```python
from build123d import *

# Parameters (mm, degrees)
SKETCH1_R           = 9.36
SKETCH1_R_2         = 7.99
EXTRUDE1_DEPTH      = 670
SKETCH2_R           = 1.5
SKETCH2_R_2         = 5.5
EXTRUDE2_DEPTH      = 10.36
EXTRUDE2_DEPTH_BACK = 10.36
SKETCH3_W           = 7
SKETCH3_H           = 22
EXTRUDE3_DEPTH      = 25
EXTRUDE3_DEPTH_BACK = 25


with BuildPart() as part:
    # Sketch1 → Extrude1 (new body)
    with BuildSketch(Plane.XY):
        Circle(SKETCH1_R)
        Circle(SKETCH1_R_2, mode=Mode.SUBTRACT)
    extrude(amount=EXTRUDE1_DEPTH)

    # Sketch2 → Extrude2 (cut, two sides)
    with BuildSketch(Plane(origin=(0, 0, 0), x_dir=(0, 0, -1), z_dir=(1, 0, 0))) as extrude2_sk:
        with Locations((-30, 0)):
            Circle(SKETCH2_R)
        with Locations((-150, 0)):
            Circle(SKETCH2_R_2)
        with Locations((-136.0625, 0)):
            Circle(SKETCH2_R)
        with Locations((-163.9375, 0)):
            Circle(SKETCH2_R)
    extrude(amount=EXTRUDE2_DEPTH, mode=Mode.SUBTRACT)
    extrude(extrude2_sk.sketch, amount=-EXTRUDE2_DEPTH_BACK, mode=Mode.SUBTRACT)

    # Sketch3 → Extrude3 (cut, two sides)
    with BuildSketch(Plane(origin=(0, 0, 0), x_dir=(1, 0, 0), z_dir=(0, 1, 0))) as extrude3_sk:
        with Locations((0, -150)):
            Rectangle(SKETCH3_W, SKETCH3_H)
    extrude(amount=EXTRUDE3_DEPTH, mode=Mode.SUBTRACT)
    extrude(extrude3_sk.sketch, amount=-EXTRUDE3_DEPTH_BACK, mode=Mode.SUBTRACT)


solid = part.part
```
The model under review builds one solid part; all positions refer to its coordinate system, in mm. Round coordinates to 2 decimals unless told otherwise and drop trailing zeros. Order: outer loops, then holes, each group sorted by start corner. A loop starts at its lowest first (then second) coordinate and runs counter-clockwise, first axis right, second up. Notation, with made-up numbers: (30.5, -21) -> (48.5, -21) arc R17 ccw to (48.5, 9) -> close; hole circle Ø7 at (14, 58). An arc over 180 degrees is marked (long way). Use a Markdown table: item, result.
Q1. We need section B-B on z = 337. Write out the cut boundary in (x, y).
Values:
| item | result |
|---|---|
| outline | circle Ø18.72 at (0, 0); hole circle Ø15.98 at (0, 0) |
Q2. For line 1 (Z direction, x = 8.35, y = 0); line 2 (X direction, y = -0.25, z = 337.5); line 3 (Y direction, x = 3.25, z = 214.5), list the stretches that pass through material, from the lowest coordinate up.
Values:
| item | result |
|---|---|
| line 1 | z = 0 to 28.5, 31.5 to 134.56, 137.56 to 144.5, 155.5 to 162.44, 165.44 to 670 |
| line 2 | x = -9.36 to -7.99, 7.99 to 9.36 |
| line 3 | y = -8.78 to -7.3, 7.3 to 8.78 |
Q3. Clearance check with flat-ended pins moving along their axes: P1, Ø4, axis at x = -3, z = 553, coming from the +Y side; P2, Ø1.6, axis at y = 7.5, z = 153.5, coming from the +X side; P3, Ø1, axis at x = 6, z = 99.5, coming from the +Y side. State where each tip first meets the part, or that it passes through.
Values:
| item | result |
|---|---|
| P1 | stops at y = 9.31 |
| P2 | stops at x = 6.54 |
| P3 | stops at y = 7.57 |
Q4. Mouldability with a two-part tool opening along Y and no side actions: class faces 1 (the cylindrical face through (-1.73, -7.8, 330.31)), 2 (the flat face through (8, 3, 0)), 3 (the cylindrical face through (-7.428, -5.695, 330.31)) as +Y half, -Y half, draft (parallel to the pull), parting line (faces both ways), or undercut.
Values:
| item | result |
|---|---|
| face 1 | undercut |
| face 2 | draft |
| face 3 | parting line |
Q5. We need section A-A on z = 150. Write out the cut boundary in (x, y).
Values:
| item | result |
|---|---|
| outline | (-7.57, -5.5) arc R9.36 ccw to (-3.5, -8.68) -> (-3.5, -7.18) arc R7.99 cw to (-5.8, -5.5) -> close; (-7.57, 5.5) -> (-5.8, 5.5) arc R7.99 cw to (-3.5, 7.18) -> (-3.5, 8.68) arc R9.36 ccw to start; (3.5, -8.68) arc R9.36 ccw to (7.57, -5.5) -> (5.8, -5.5) arc R7.99 cw to (3.5, -7.18) -> close; (3.5, 7.18) arc R7.99 cw to (5.8, 5.5) -> (7.57, 5.5) arc R9.36 ccw to (3.5, 8.68) -> close |
